Here's how the part is built. I have some questions about the finished solid (model axes, mm). A direction names the side the tool comes from. Round coordinates to 2 decimals unless told otherwise and drop trailing zeros. Loops run counter-clockwise (first coordinate to the right, second up) from the corner with the lowest first, then second, coordinate; pieces in that order, holes last. Notation, with made-up numbers: M -27.75,-7.75 L 6.25,-7.75 A7 cw 6.25,5.25 Z; hole C -2.75,-25 d2. An arc over 180 degrees is marked long. Answer as a JSON object with one key per item and string values.
from build123d import *

# Parameters (mm, degrees)
F1_DEPTH  = 36
F2_W      = 22
F2_H      = 70.056442
F3_DEPTH  = 6
F4_R      = 12
F5_DEPTH  = 143.057441
F6_R      = 30
F7_DEPTH  = 12
F8_W      = 12
F8_H      = 36
F9_W      = 12
F9_H      = 36
F12_DEPTH = 25


with BuildPart() as f1:
    # F0 (on Right) → F1 (new body, symmetric)
    with BuildSketch(Plane.YZ):
        Polygon((-54.158381, 45.637498), (-90.158381, 45.637498), (-90.158381, -38.362502), (-20.101939, -38.362502), (-20.101939, -44.362502), (52.898061, -44.362502), (52.898061, -19.362502), (-54.158381, -19.362502), align=None)
    extrude(amount=F1_DEPTH, both=True)

    # F2 (on face) → F3 (join)
    with BuildSketch(Plane(origin=(0, 0, -38.362502), x_dir=(1, 0, 0), z_dir=(0, 0, -1))):
        with Locations((-25, 55.13016)):
            Rectangle(F2_W, F2_H)
    extrude(amount=F3_DEPTH)

    # F4 (on face) → F5 (cut, through all)
    with BuildSketch(Plane.XZ.offset(90.158381)):
        with Locations((0, 3.637498)):
            Circle(F4_R)
    extrude(amount=-F5_DEPTH, mode=Mode.SUBTRACT)

    # F6 (on face) → F7 (cut)
    with BuildSketch(Plane.XZ.offset(90.158381)):
        with Locations((0, 3.637498)):
            Circle(F6_R)
    extrude(amount=-F7_DEPTH, mode=Mode.SUBTRACT)

    # F8 (on face) → F10 section 0
    with BuildSketch(Plane.YZ.offset(36)):
        with Locations((-84.158381, 3.637498)):
            Rectangle(F8_W, F8_H)
    # F9 (on face) → F10 section 1
    with BuildSketch(Plane(origin=(-36, 0, 0), x_dir=(0, -1, 0), z_dir=(-1, 0, 0))):
        with Locations((84.158381, 3.637498)):
            Rectangle(F9_W, F9_H)
    loft(mode=Mode.SUBTRACT)

    # F11 (on face) → F12 (cut)
    with BuildSketch(Plane.XY.offset(-19.362502)):
        with BuildLine():
            Line((12, 2.898061), (12, 52.898061))
            Line((12, 52.898061), (-12, 52.898061))
            Line((-12, 52.898061), (-12, 2.898061))
            ThreePointArc((-12, 2.898061), (0, -9.101939), (12, 2.898061))
        make_face()
    extrude(amount=-F12_DEPTH, mode=Mode.SUBTRACT)


solid = f1.part
Item 1: I want a section at A-A on y = 24.5. List the corners of the cut face in (x, z) for me, plus the area to 3 significant figures.
Solution:
{"outline": "M -36,-44.36 L -12,-44.36 L -12,-19.36 L -36,-19.36 Z; M 12,-44.36 L 36,-44.36 L 36,-19.36 L 12,-19.36 Z", "area": "1,200 mm2"}
Item 2: I want a section at C-C on z = 14. List the corners of the cut face in (x, y) for me, plus the area to 3 significant figures.
Solution:
{"outline": "M -36,-78.16 L -6.05,-78.16 L -6.05,-54.16 L -36,-54.16 Z; M 6.05,-78.16 L 36,-78.16 L 36,-54.16 L 6.05,-54.16 Z", "area": "1,440 mm2"}
Item 3: I want a section at D-D on x = -27. List the corners of the cut face in (y, z) for me, plus the area to 3 significant figures.
Solution:
{"outline": "M -90.16,-44.36 L 52.9,-44.36 L 52.9,-19.36 L -54.16,-19.36 L -54.16,45.64 L -90.16,45.64 L -90.16,21.64 L -78.16,21.64 L -78.16,-14.36 L -90.16,-14.36 Z", "area": "5,480 mm2"}
Item 4: For P1, Ø1.5, axis at x = 13, z = 19, coming from the +Y side; P2, Ø6.5, axis at y = -72, z = -41, coming from the +X side; P3, Ø25, axis at x = 9, y = -48.5, coming from the -Z side; P4, Ø3, axis at x = 10.5, z = -42, coming from the -Y side, each with a flat end and sliding along its axis, tell me the tip position at first contact or that it passes through.
Solution:
{"P1": "stops at y = -54.16", "P2": "stops at x = 36", "P3": "stops at z = -38.36", "P4": "stops at y = -20.1"}
Item 5: For faces 4 (the face through (0.389, -84.242, 33.635)), 5 (the face through (12, 28, -32)), 6 (the face through (-30, -84, -14.363)), which set-ups out of +Z, -Z, +X, -X, +Y, -Y let a thin tool reach every point of the face, with its end or its side?
Solution:
{"face 4": "-Y", "face 5": "+Z, -Z, +Y", "face 6": "+X, -X, -Y"}
Item 6: We'd pull the mould along Z, two halves only. Please class faces 1 (the face through (1, -72, 45.637)), 2 (the face through (-8.5, -19.6, -44.363)), 3 (the face through (30, -84, 21.637)): +Z half, -Z half, draft (parallel to the pull), parting line (faces both ways), or undercut.
Solution:
{"face 1": "+Z half", "face 2": "-Z half", "face 3": "undercut"}
Item 7: I want a section at B-B on x = 0. List the corners of the cut face in (y, z) for me.
Solution:
{"outline": "M -90.16,-38.36 L -20.1,-38.36 L -20.1,-44.36 L -9.1,-44.36 L -9.1,-19.36 L -54.16,-19.36 L -54.16,-8.36 L -78.16,-8.36 L -78.16,-26.36 L -90.16,-26.36 Z; M -90.16,33.64 L -78.16,33.64 L -78.16,15.64 L -54.16,15.64 L -54.16,45.64 L -90.16,45.64 Z"}
Item 8: If I drill on L1, parallel to Z at x = 0, y = -62.25; L2, parallel to Y at x = -22.5, z = 30; L3, parallel to Y at x = 16.5, z = -8, over which ranges is the centre line in solid material (lowest first)? Write a range as from..to.
Solution:
{"L1": "z = -38.36..-8.36, 15.64..45.64", "L2": "y = -90.16..-54.16", "L3": "y = -78.16..-54.16"}
